The listing builds one solid part. Answer for the finished solid, in the listing's coordinates (mm). Face numbers are marked on the shaded views. A direction names the side the tool comes from. Round coordinates to 2 decimals unless told otherwise and drop trailing zeros. Loops run counter-clockwise (first coordinate to the right, second up) from the corner with the lowest first, then second, coordinate; pieces in that order, holes last. Notation, with made-up numbers: (30.25, 37.5) - (82.25, 37.5) arc R18 ccw to (82.25, 55.5) - close; hole circle Ø11 at (68.25, 32). An arc over 180 degrees is marked (long way). Write item = value, one per line. Start each with the question number.
1) A tool of negligible diameter and unlimited length cuts with its end or side. For the marked faces 4, 5 and 6, from which of +Z, -Z, +X, -X, +Y, -Y can it reach the whole face along a straight path? Write none if from no direction.
2) Section A-A, the plane x = 22 is taken. Determine the outline of the cut face in (y, z).
3) Given pin 1 Ø2 at (x, z) = (24.5, 19.5) entering from +Y; pin 2 Ø8 at (x, z) = (8.5, -5) entering from -Y; pin 3 Ø6 at (x, y) = (-1, -10.5) entering from -Z; pin 4 Ø5 at (y, z) = (-9.5, 8) entering from +X, each flat-ended and moving along its own axis, determine where each tip first touches the part or whether it passes through.
4) Section D-D, the plane y = -5.5 is taken. Determine the outline of the cut face in (x, z), and give its area (3 significant figures).
5) Section B-B, the plane z = 7.5 is taken. Determine the outline of the cut face in (x, y), and give its area (3 significant figures).
6) Section C-C, the plane z = 13.4 is taken. Determine the outline of the cut face in (x, y).
7) Straight lines are drawn through the part: line 1 along Z through (x, y) = (0, -1.9); line 2 along Z through (x, y) = (-24.5, -1.05); line 3 along Y through (x, z) = (0, 22.5). For each, find the intervals that lie inside material, in ascending order.
8) For a pull along X with two mould halves and no side action, classify the marked faces 1, 2 and 3 as released by +X, released by -X, zero draft, split by the parting line, or undercut.
from build123d import *

# Parameters (mm, degrees)
F0_W      = 63.5
F0_H      = 50.8
F0_R      = 4.25
F1_DEPTH  = 3
F2_W      = 17
F2_H      = 32
F3_DEPTH  = 3.001
F4_R      = 5
F5_W      = 15
F5_H      = 24
F5_R      = 4.25
F6_DEPTH  = 10
F8_D      = 4.2
F9_R      = 4
F10_R     = 4
F11_DEPTH = 3.0010001
F12_R     = 1.25
F13_DEPTH = 13.0010001
F14_R     = 1


with BuildPart() as f1:
    # F0 (on Front) → F1 (new body)
    with BuildSketch(Plane.XZ):
        Rectangle(F0_W, F0_H)
        with Locations((0, 13.4)):
            Circle(F0_R, mode=Mode.SUBTRACT)
    extrude(amount=F1_DEPTH)

    # F2 (on face) → F3 (cut, through all)
    with BuildSketch(Plane.XZ.offset(3)):
        with Locations((20.25, 0)):
            Rectangle(F2_W, F2_H)
        with Locations((-20.25, 0)):
            Rectangle(F2_W, F2_H)
    extrude(amount=-F3_DEPTH, mode=Mode.SUBTRACT)

    # F4
    f4_edges = [f1.edges().sort_by_distance(p)[0] for p in [
        (-31.75, -1.5, 25.4),
        (31.75, -1.5, 25.4),
        (31.75, -1.5, -25.4),
        (-31.75, -1.5, -25.4),
    ]]
    fillet(f4_edges, radius=F4_R)

    # F5 (on face) → F6 (join)
    with BuildSketch(Plane.XZ.offset(3)):
        with Locations((0, 13.4)):
            Rectangle(F5_W, F5_H)
        with Locations((0, 13.4)):
            Circle(F5_R, mode=Mode.SUBTRACT)
    extrude(amount=F6_DEPTH)

    # F8 (through all)
    with Locations(Plane.XY.offset(25.4)):
        with Locations((0, -6.5)):
            Hole(F8_D / 2)

    # F9
    f9_edges = [f1.edges().sort_by_distance(p)[0] for p in [
        (-7.5, -8, 1.4),
        (7.5, -8, 1.4),
        (7.5, -8, 25.4),
        (-7.5, -8, 25.4),
    ]]
    fillet(f9_edges, radius=F9_R)

    # F10 (on face) → F11 (cut, through all)
    with BuildSketch(Plane.XZ.offset(3)):
        with Locations((0, -5.4962742142)):
            Circle(F10_R)
        with Locations((0, -18.0155653507)):
            Circle(F10_R)
    extrude(amount=-F11_DEPTH, mode=Mode.SUBTRACT)

    # F12 (on face) → F13 (cut, through all)
    with BuildSketch(Plane(origin=(0, 0, 0), x_dir=(-1, 0, 0), z_dir=(0, 1, 0))):
        with Locations((-24.5, 19.5)):
            Circle(F12_R)
        with Locations((-16, 19.5)):
            Circle(F12_R)
        with Locations((16, 19.5)):
            Circle(F12_R)
        with Locations((24.5, 19.5)):
            Circle(F12_R)
        with Locations((-24.5, -19.5)):
            Circle(F12_R)
        with Locations((-16, -19.5)):
            Circle(F12_R)
        with Locations((16, -19.5)):
            Circle(F12_R)
        with Locations((24.5, -19.5)):
            Circle(F12_R)
    extrude(amount=-F13_DEPTH, mode=Mode.SUBTRACT)

    # F14
    f14_edges = [f1.edges().sort_by_distance(p)[0] for p in [
        (28.75, -1.5, 16),
        (-11.75, -1.5, 16),
        (11.75, -1.5, 16),
        (-28.75, -1.5, 16),
        (-28.75, -1.5, -16),
        (11.75, -1.5, -16),
        (-11.75, -1.5, -16),
        (28.75, -1.5, -16),
    ]]
    fillet(f14_edges, radius=F14_R)


solid = f1.part
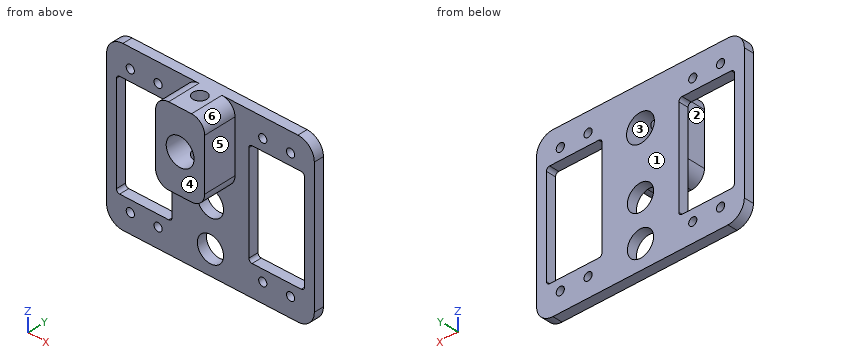
Geometry check:
q1.face_4 = +Z, -Z, +X, -X, -Y
q1.face_5 = +Z, -Z, +X, -Y
q1.face_6 = +Z, +X, -Y
q2.outline = (-3, -25.4) - (0, -25.4) - (0, -16) - (-3, -16) - close; (-3, 16) - (0, 16) - (0, 25.4) - (-3, 25.4) - close
q3.pin_1 = through
q3.pin_2 = -3
q3.pin_3 = 1.4
q3.pin_4 = 7.5
q4.outline = (-7.5, 5.4) arc R4 ccw to (-3.5, 1.4) - (-1.85, 1.4) - (-1.85, 9.57) arc R4.25 cw to (-1.85, 17.23) - (-1.85, 25.4) - (-3.5, 25.4) arc R4 ccw to (-7.5, 21.4) - close; (1.85, 1.4) - (3.5, 1.4) arc R4 ccw to (7.5, 5.4) - (7.5, 21.4) arc R4 ccw to (3.5, 25.4) - (1.85, 25.4) - (1.85, 17.23) arc R4.25 cw to (1.85, 9.57) - close
q4.area = 231 mm2
q5.outline = (-31.75, -3) - (-28.75, -3) - (-28.75, 0) - (-31.75, 0) - close; (-11.75, -3) - (-7.5, -3) - (-7.5, -13) - (7.5, -13) - (7.5, -3) - (11.75, -3) - (11.75, 0) - (-11.75, 0) - close; (28.75, -3) - (31.75, -3) - (31.75, 0) - (28.75, 0) - close; hole circle Ø4.2 at (0, -6.5)
q5.area = 225 mm2
q6.outline = (-31.75, -3) - (-28.75, -3) - (-28.75, 0) - (-31.75, 0) - close; (-11.75, -3) - (-7.5, -3) - (-7.5, -13) - (-4.25, -13) - (-4.25, 0) - (-11.75, 0) - close; (4.25, -13) - (7.5, -13) - (7.5, -3) - (11.75, -3) - (11.75, 0) - (4.25, 0) - close; (28.75, -3) - (31.75, -3) - (31.75, 0) - (28.75, 0) - close
q7.line_1 = -25.4 to -22.02, -14.02 to -9.5, -1.5 to 9.15, 17.65 to 25.4
q7.line_2 = -25.4 to -20.75, -18.25 to -16, 16 to 18.25, 20.75 to 25.4
q7.line_3 = -13 to -8.6, -4.4 to 0
q8.face_1 = zero draft
q8.face_2 = released by -X
q8.face_3 = undercut
